Autodesk Inventor part; units mm, degrees
ref_plane "Work Plane2" through (0, 19.05, 0) normal (0, 1, 0) x (1, 0, 0)
ref_plane "Work Plane1" through (0, 19.05, 0) normal (0, 1, 0) x (1, 0, 0)
ref_plane "YZ Plane" through (0, 0, 0) normal (1, 0, 0) x (0, 1, 0)
sketch "Sketch1" plane through (0, 0, 0) normal (0, 1, 0) x (-1, 0, 0)
  circle A0 centre (0, 0) radius 8.0645
  circle A1 centre (0, -63.5) radius 6.985
  circle A2 centre (0, 63.5) radius 6.985
  line L0 (-39.6048, 88.9) -> (39.6048, 88.9)
  line L1 (39.6048, 88.9) -> (39.6048, -88.9)
  line L2 (39.6048, -88.9) -> (-39.6048, -88.9)
  line L3 (-39.6048, -88.9) -> (-39.6048, 88.9)
  line L4 (-39.6048, 88.9) -> (39.6048, -88.9) construction
  line L5 (39.6048, 88.9) -> (-39.6048, -88.9) construction
  line L6 (10.9754, 63.5) -> (10.9754, 0) construction
  point P0 (0, 0)
  point P1 (0, 0)
  point P2 (0, 63.5)
  dimension "d0" = 16.129
  dimension "d1" = 13.97
  dimension "d2" = 13.97
  dimension "d28" = 177.8
  dimension "d30" = 25.4
  dimension "d31" = 25.4
extrude "Extrusion4" add sketch "Sketch1" along normal blind 19.05
ref_plane "Work Plane2" through (0, 19.05, 0) normal (0, 1, 0) x (1, 0, 0)
sketch "Sketch2" plane through (0, 19.05, 0) normal (0, 1, 0) x (1, 0, 0)
  circle A0 centre (-11.2395, 0) radius 1.25
  circle A1 centre (0, 0) radius 7.94
  circle A2 centre (5.6197, -9.7337) radius 1.25
  circle A3 centre (5.6198, 9.7337) radius 1.25
  dimension "d11" = 2.5
  dimension "d12" = 11.2395
  dimension "d15" = 360
ref_plane "Work Plane1" through (0, 19.05, 0) normal (0, 1, 0) x (1, 0, 0)
extrude "Extrusion5" cut sketch "Sketch2" against normal up to next contours A0 | A2 | A3
sketch "Sketch6" plane through (0, 19.05, 0) normal (0, 1, 0) x (1, 0, 0)
  line L0 (0, -38.1) -> (0, -18.8395)
  line L1 (0, 18.8395) -> (0, 38.1)
  line L2 (39.6048, 88.9) -> (-39.6048, 88.9)
  line L3 (0, 88.9) -> (-39.6048, 88.9)
  line L4 (-39.6048, -88.9) -> (39.6048, -88.9)
  line L5 (-39.6048, 88.9) -> (-39.6048, -88.9)
  line L6 (-39.6048, -88.9) -> (0, -88.9)
  circle A0 centre (0, 0) radius 8.0645
  arc A1 (0, 18.8395) -> (0, -18.8395) centre (0, 0) ccw
  arc A2 (0, -50.8) -> (0, -76.2) centre (0, -63.5) ccw
  line L7 (0, -38.1) -> (0, -50.8)
  line L8 (0, -76.2) -> (0, -88.9)
  arc A3 (0, 76.2) -> (0, 50.8) centre (0, 63.5) ccw
  line L9 (0, 88.9) -> (0, 76.2)
  line L10 (0, 50.8) -> (0, 38.1)
  circle A4 centre (0, 63.5) radius 6.477
  circle A5 centre (0, -63.5) radius 6.477
  circle A6 centre (-11.2395, 0) radius 1.25
  point P0 (0, 0)
  dimension "d41" = 25.4
  dimension "d42" = 25.4
  dimension "d44" = 12.954
  dimension "d45" = 12.954
  dimension "d77" = 6.35
extrude "Extrusion6" cut sketch "Sketch6" against normal blind 19.05 contours L7 A2 L8 L4 L5 L2 L9 A3 L10 L1 A1 L0
fillet "Fillet5" radius 12.7 4 edges at (0, 9.525, 50.8) (0, 9.525, -50.8) (0, 9.525, -18.8395) (0, 9.525, 18.8395)
sketch "Sketch8" plane through (0, 19.05, -88.9) normal (-1, 0, 0) x (0, 0, 1)
  line L0 (33.355, -16.3528) -> (33.355, -2.5052)
  line L1 (15.575, -2.511) -> (15.575, -16.351)
  line L2 (27.5747, -16.3528) -> (27.5747, -2.5052)
  line L3 (21.1759, -16.351) -> (21.1759, -2.511)
  line L4 (33.355, -16.3528) -> (27.5747, -16.3528)
  line L5 (33.355, -2.5052) -> (27.5747, -2.5052)
  line L6 (15.575, -16.351) -> (21.1759, -16.351)
  line L7 (21.1759, -2.511) -> (15.575, -2.511)
  point P0 (88.9, -19.05)
extrude "Extrusion7" cut sketch "Sketch8" along normal up to next
mirror "Mirror1" about plane through (0, 0, 0) normal (0, 0, 1) of "Extrusion7"
fillet "Fillet6" radius 12.7 2 edges at (0, 9.525, 88.9) (0, 9.525, -88.9)
sketch "Sketch12" plane through (0, 19.05, 0) normal (0, 1, 0) x (1, 0, 0)
  line L0 (39.6048, -88.9) -> (39.6048, 88.9)
  line L1 (39.6048, -82.55) -> (19.685, -82.55)
  line L2 (19.685, -82.55) -> (19.685, 82.55)
  line L3 (19.685, 82.55) -> (39.6048, 82.55)
  line L4 (39.6048, 82.55) -> (39.6048, -82.55)
  line L5 (39.6048, 88.9) -> (12.7, 88.9)
  line L6 (12.7, -88.9) -> (39.6048, -88.9)
  circle A0 centre (0, -63.5) radius 6.985
  point P0 (0, 0)
  dimension "d72" = 6.35
  dimension "d73" = 6.35
  dimension "d74" = 12.7
extrude "Extrusion10" cut sketch "Sketch12" against normal up to next contours L1 L2 L3 L0
sketch "Sketch13" plane through (39.6048, 0, 88.9) normal (1, 0, 0) x (0, 0, -1)
  line L0 (0, 0) -> (0, 19.05)
  line L1 (171.45, 0) -> (6.35, 0)
  line L2 (0, 19.05) -> (6.35, 19.05)
  line L3 (6.35, 19.05) -> (6.35, 0)
  line L4 (6.35, 0) -> (0, 0)
  line L5 (0, 0) -> (0, 19.05)
  line L6 (171.45, 19.05) -> (171.45, 0)
  line L7 (177.8, 19.05) -> (177.8, 0)
  line L8 (171.45, 19.05) -> (177.8, 19.05)
  line L9 (177.8, 19.05) -> (177.8, 0)
  line L10 (177.8, 0) -> (171.45, 0)
  line L11 (171.45, 0) -> (171.45, 19.05)
  point P0 (88.9, 0)
extrude "Extrusion11" add sketch "Sketch13" along normal blind 50.8
sketch "Sketch14" plane through (19.685, 19.05, 82.55) normal (1, 0, 0) x (0, 0, -1)
  line L0 (0, -19.05) -> (0, 0)
  line L1 (0, 0) -> (165.1, 0)
  line L2 (165.1, 0) -> (165.1, -19.05)
  line L3 (165.1, -19.05) -> (0, -19.05)
  point P0 (82.55, -19.05)
extrude "Extrusion12" add sketch "Sketch14" along normal blind 6.35
properties part number "AlteredPlatformATEdit"
Can you work these out from the model? Positions are in its coordinate system, mm. A direction names the side the tool comes from. Round coordinates to 2 decimals unless told otherwise and drop trailing zeros. Loops run counter-clockwise (first coordinate to the right, second up) from the corner with the lowest first, then second, coordinate; pieces in that order, holes last. Notation, with made-up numbers: (42, 57) - (74, 57) arc R35 cw to (74, 91) - close; hole circle Ø6 at (64, 7.25). An arc over 180 degrees is marked (long way). Write item = value, one per line. Start each with the question number.
(1) For P1, Ø3, axis at x = -6.5, y = 12, coming from the -Z side; P2, Ø1.8, axis at x = -9.5, y = 10, coming from the -Z side; P3, Ø1, axis at y = 11, z = -49, coming from the +X side (3 decimals); P4, Ø11, axis at x = 0, z = 63.5, coming from the +Y side, each with a flat end and sliding along its axis, tell me the tip position at first contact or that it passes through.
(2) If we section it at D-D (z = 36): Please give me the cut outline in (x, y) (3 decimals), and give its area (3 significant figures).
(3) If we section it at A-A (z = -63.5): Please give me the cut outline in (x, y) (3 decimals), and give its area (3 significant figures).
(4) If we mould it in two halves opening along Z, with no side actions, what happens to faces 6 (the face through (-10, 10, 61.325)), 7 (the face through (19, 19.05, 0)), 8 (the face through (3.62, 9.39, -85.08))? For each: released by +Z, released by -Z, zero draft, split by the parting line, or undercut.
(5) If I drill on probe 1 along Z at (x, y) = (73.5, 14.75); probe 2 along X at (y, z) = (6.75, 73) (3 decimals); probe 3 along Z at (x, y) = (-4.5, 12.25) (3 decimals), over which ranges is the centre line in solid material (lowest first)? Write a range as [from, to].
(6) If we section it at C-C (x = 2): Please give me the cut outline in (y, z).
(7) For faces 1 (the face through (-9, 10, 67.724)), 2 (the face through (90.405, 10, -86)), 3 (the face through (51, 9, -88.9)), 4 (the face through (0, 10, 35)), 5 (the face through (59, 10, 82.55)), which set-ups out of +Z, -Z, +X, -X, +Y, -Y let a thin tool reach every point of the face, with its end or its side?
(8) If we section it at B-B (x = 61): Please give me the cut outline in (y, z).
Ans:
q1.P1 = -75.17
q1.P2 = -67.72
q1.P3 = 26.035
q1.P4 = through
q2.outline = (0, 0) - (26.035, 0) - (26.035, 19.05) - (0, 19.05) - close
q2.area = 496 mm²
q3.outline = (-12.7, 0) - (-6.985, 0) - (-6.985, 19.05) - (-12.7, 19.05) - close; (6.985, 0) - (26.035, 0) - (26.035, 19.05) - (6.985, 19.05) - close
q3.area = 472 mm²
q4.face_6 = undercut
q4.face_7 = zero draft
q4.face_8 = released by -Z
q5.probe_1 = [-88.9, -82.55], [82.55, 88.9]
q5.probe_2 = [0, 26.035]
q5.probe_3 = [-75.376, -73.325], [-55.545, -51.201], [-19.172, -6.692], [6.692, 19.172], [51.201, 55.545], [73.325, 75.376]
q6.outline = (0, -83.04) - (19.05, -83.04) - (19.05, -70.19) - (0, -70.19) - close; (0, -56.81) - (19.05, -56.81) - (19.05, -7.81) - (0, -7.81) - close; (0, 7.81) - (19.05, 7.81) - (19.05, 56.81) - (0, 56.81) - close; (0, 70.19) - (19.05, 70.19) - (19.05, 83.04) - (0, 83.04) - close
q7.face_1 = -X
q7.face_2 = +Z, -Z, +X, +Y, -Y
q7.face_3 = -Z, +X, -X, +Y, -Y
q7.face_4 = -X, +Y, -Y
q7.face_5 = +X, +Y, -Y
q8.outline = (0, -88.9) - (19.05, -88.9) - (19.05, -82.55) - (0, -82.55) - close; (0, 82.55) - (19.05, 82.55) - (19.05, 88.9) - (0, 88.9) - close
